```python
from build123d import *

# Parameters (mm, degrees)
EXTRUDE_THIN1_DEPTH            = 100
F_5_0MM_DOWEL_HOLE1_AT_2_COUNT = 2
F_5_0MM_DOWEL_HOLE1_AT_2_PITCH = 150
F_5_0MM_DOWEL_HOLE2_AT_2_COUNT = 2
F_5_0MM_DOWEL_HOLE2_AT_2_PITCH = 150


with BuildPart() as part:
    # Sketch2 → Extrude-Thin1 (new, symmetric)
    with BuildSketch(Plane(origin=(0, 0, 0), x_dir=(0, 0, -1), z_dir=(1, 0, 0))):
        Polygon((0, 50), (0, 0), (50, 0), (50, 5), (5, 5), (5, 50), align=None)
    extrude(amount=EXTRUDE_THIN1_DEPTH, both=True)

    # Sketch5 → Ø5.0mm Dowel Hole1 (revolve, cut)
    with BuildSketch(Plane(origin=(75, 25, -5), x_dir=(0, 1, 0), z_dir=(1, 0, 0))):
        Polygon((0, 0), (0, 5), (2.525, 5), (2.5, 4.975), (2.5, 0), align=None)
    f_5_0mm_dowel_hole1 = revolve(axis=Axis((75, 25, -11.35), (0, 0, 1)), mode=Mode.SUBTRACT)

    # Ø5.0mm Dowel Hole1 at 2: Ø5.0mm Dowel Hole1 ×2
    with Locations(*[(-i * F_5_0MM_DOWEL_HOLE1_AT_2_PITCH, 0, 0) for i in range(1, F_5_0MM_DOWEL_HOLE1_AT_2_COUNT)]):
        add(f_5_0mm_dowel_hole1, mode=Mode.SUBTRACT)

    # Sketch7 → Ø5.0mm Dowel Hole2 (revolve, cut)
    with BuildSketch(Plane(origin=(-75, 5, -25), x_dir=(0, 0, 1), z_dir=(1, 0, 0))):
        Polygon((0, 0), (0, 5), (2.525, 5), (2.5, 4.975), (2.5, 0), align=None)
    f_5_0mm_dowel_hole2 = revolve(axis=Axis((-75, 11.35, -25), (0, -1, 0)), mode=Mode.SUBTRACT)

    # Ø5.0mm Dowel Hole2 at 2: Ø5.0mm Dowel Hole2 ×2
    with Locations(*[(i * F_5_0MM_DOWEL_HOLE2_AT_2_PITCH, 0, 0) for i in range(1, F_5_0MM_DOWEL_HOLE2_AT_2_COUNT)]):
        add(f_5_0mm_dowel_hole2, mode=Mode.SUBTRACT)


solid = part.part
```
The model under review builds one solid part; all positions refer to its coordinate system, in mm. A direction names the side the tool comes from. Round coordinates to 2 decimals unless told otherwise and drop trailing zeros. Write each loop counter-clockwise with the first axis right and the second up, starting at its lowest first coordinate (ties: lowest second). Pieces come first, ordered by that corner, then holes. Notation, with made-up numbers: (-3, -20) - (28, -20) arc R12 cw to (28, 1) - close; hole circle Ø4 at (85, -23). An arc over 180 degrees is marked (long way). One line per question, with ' | ' between items.
Item 1: Add section C-C, the plane y = 25. Give the boundary of the cut face in (x, z) (3 decimals), then the cut area to 3 significant figures.
Resolved:
outline: (-100, -5) - (-77.5, -5) - (-77.5, -0.025) - (-77.525, 0) - (-100, 0) - close; (-72.5, -5) - (72.5, -5) - (72.5, -0.025) - (72.475, 0) - (-72.475, 0) - (-72.5, -0.025) - close; (77.5, -5) - (100, -5) - (100, 0) - (77.525, 0) - (77.5, -0.025) - close | area: 950 mm2
Item 2: To check wall thickness, follow probe 1 along X at (y, z) = (2.05, -25); probe 2 along Y at (x, z) = (75, -3.55); probe 3 along X at (y, z) = (4.5, -26.5). State the ranges of each line that lie inside material, in increasing order.
Resolved:
probe 1: x = -100 to -77.5, -72.5 to 72.5, 77.5 to 100 | probe 2: y = 0 to 22.5, 27.5 to 50 | probe 3: x = -100 to -77, -73 to 73, 77 to 100
Item 3: The part is to be moulded in two halves that separate along Z. For faces 3 (the face through (77.44, 2.55, -25.54)), 4 (the face through (1, 27, -5)), 5 (the face through (-72.56, 24.46, -2.55)), say which applies: pulls with the +Z half, pulls with the -Z half, needs draft (parallel to the pull), parting line crosses it, or undercut.
Resolved:
face 3: undercut | face 4: pulls with the -Z half | face 5: needs draft
Item 4: Add section D-D, the plane x = -63. Give the boundary of the cut face in (y, z), then the cut area to 3 significant figures.
Resolved:
outline: (0, -50) - (5, -50) - (5, -5) - (50, -5) - (50, 0) - (0, 0) - close | area: 475 mm2
Item 5: Add section B-B, the plane z = -25. Give the boundary of the cut face in (x, y) (3 decimals).
Resolved:
outline: (-100, 0) - (-77.525, 0) - (-77.5, 0.025) - (-77.5, 5) - (-100, 5) - close; (-72.5, 0.025) - (-72.475, 0) - (72.475, 0) - (72.5, 0.025) - (72.5, 5) - (-72.5, 5) - close; (77.5, 0.025) - (77.525, 0) - (100, 0) - (100, 5) - (77.5, 5) - close
Item 6: For faces 1 (the face through (1, 5, -28)), 2 (the face through (1, 25, 0)), list the 3-axis set-ups (+Z, -Z, +X, -X, +Y, -Y) from which the entire face can be reached by the end or side of a thin tool; tool diameter is ignored.
Resolved:
face 1: -Z, +X, -X, +Y | face 2: +Z, +X, -X, +Y, -Y
Item 7: For P1, Ø8, axis at x = 75, y = 25, coming from the +Z side; P2, Ø6, axis at y = 9, z = -26.5, coming from the -X side; P3, Ø6, axis at x = -7.5, y = 39.5, coming from the -Z side; P4, Ø6.5, axis at x = -75, z = -25, coming from the +Y side, all flat-tipped, find the tip position at first contact; note any pin that passes through.
Resolved:
P1: stops at z = 0 | P2: passes through | P3: stops at z = -5 | P4: stops at y = 5
Item 8: Add section A-A, the plane x = 75. Give the boundary of the cut face in (y, z) (3 decimals).
Resolved:
outline: (0, -50) - (5, -50) - (5, -27.5) - (0.025, -27.5) - (0, -27.525) - close; (0, -22.475) - (0.025, -22.5) - (5, -22.5) - (5, -5) - (22.5, -5) - (22.5, -0.025) - (22.475, 0) - (0, 0) - close; (27.5, -5) - (50, -5) - (50, 0) - (27.525, 0) - (27.5, -0.025) - close
